Input: part model. Units: mm. Frame: model coordinates. Face numbers are marked on the shaded views. A direction names the side the tool comes from. Round coordinates to 2 decimals unless told otherwise and drop trailing zeros. Loops run counter-clockwise (first coordinate to the right, second up) from the corner with the lowest first, then second, coordinate; pieces in that order, holes last. Notation, with made-up numbers: (-35.75, 37.25) -> (21.25, 37.25) arc R30 cw to (21.25, 73.25) -> close; hole circle Ø8 at (76, -17). An arc over 180 degrees is marked (long way). Answer as a JSON object with one key per item and string values.
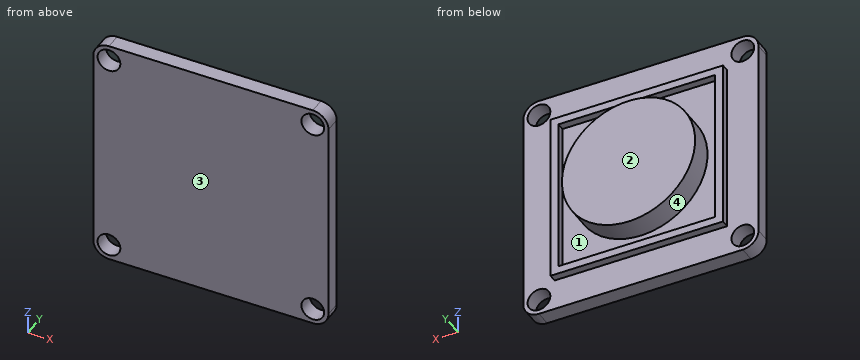
Autodesk Inventor part; units mm, degrees
ref_plane "YZ Plane" through (0, 0, 0) normal (1, 0, 0) x (0, 1, 0)
ref_plane "XZ Plane" through (0, 0, 0) normal (0, 1, 0) x (-1, 0, 0)
ref_plane "XY Plane" through (0, 0, 0) normal (0, 0, 1) x (1, 0, 0)
sketch "Boceto1" plane through (0, 0, 0) normal (0, 1, 0) x (-1, 0, 0)
  line L0 (-13, 15) -> (13, 15)
  line L1 (15, 13) -> (15, -13)
  line L2 (13, -15) -> (-13, -15)
  line L3 (-15, -13) -> (-15, 13)
  line L4 (-15, 15) -> (15, -15) construction
  line L5 (15, 15) -> (-15, -15) construction
  arc A0 (13, -15) -> (15, -13) centre (13, -13) ccw
  arc A1 (15, 13) -> (13, 15) centre (13, 13) ccw
  arc A2 (-13, 15) -> (-15, 13) centre (-13, 13) ccw
  arc A3 (-15, -13) -> (-13, -15) centre (-13, -13) ccw
  point P0 (0, 0)
  dimension "d0" = 30
  dimension "d1" = 30
  dimension "d2" = 2
extrude "Extrusión1" add sketch "Boceto1" along normal blind 2
sketch "Boceto2" plane through (0, 2, 0) normal (0, 1, 0) x (1, 0, 0)
  circle A0 centre (0, 0) radius 8.5
  dimension "d5" = 17
extrude "Extrusión2" add sketch "Boceto2" along normal blind 3
sketch "Boceto3" plane through (0, 2, 0) normal (0, 1, 0) x (1, 0, 0)
  line L0 (10, -10) -> (-10, -10)
  line L1 (-10, -10) -> (-10, 10)
  line L2 (-10, 10) -> (10, 10)
  line L3 (10, 10) -> (10, -10)
  line L4 (10, -10) -> (-10, 10) construction
  line L5 (-10, -10) -> (10, 10) construction
  line L6 (11, -11) -> (-11, -11)
  line L7 (-11, -11) -> (-11, 11)
  line L8 (-11, 11) -> (11, 11)
  line L9 (11, 11) -> (11, -11)
  line L10 (11, -11) -> (-11, 11) construction
  line L11 (-11, -11) -> (11, 11) construction
  point P0 (0, 0)
  dimension "d8" = 1
  dimension "d9" = 1
  dimension "d10" = 10
  dimension "d11" = 10
extrude "Extrusión3" add sketch "Boceto3" along normal blind 1
sketch "Boceto4" plane through (0, 0, 0) normal (0, -1, 0) x (1, 0, 0)
  point P0 (13, -13)
  point P1 (-13, -13)
hole "Agujero1" at (13, 0, -13) at (-13, 0, -13) direction (0, 1, 0) diameter 2.9 end through all
sketch "Boceto5" plane through (0, 0, 0) normal (0, -1, 0) x (1, 0, 0)
  point P0 (-13, 13)
hole "Agujero2" at (-13, 0, 13) direction (0, 1, 0) diameter 2.9 end through all
sketch "Boceto6" plane through (0, 0, 0) normal (0, -1, 0) x (1, 0, 0)
  point P0 (13, 13)
hole "Agujero3" at (13, 0, 13) direction (0, 1, 0) diameter 2.9 end through all
properties part number "Tapa trasera" material "Plástico PET"
1) Section C-C, the plane z = 0. Output: boundary loops of the cut face in (x, y).
Output:
{"outline": "(-15, 0) -> (15, 0) -> (15, 2) -> (11, 2) -> (11, 3) -> (10, 3) -> (10, 2) -> (8.5, 2) -> (8.5, 5) -> (-8.5, 5) -> (-8.5, 2) -> (-10, 2) -> (-10, 3) -> (-11, 3) -> (-11, 2) -> (-15, 2) -> close"}
2) Section B-B, the plane x = 0. Output: boundary loops of the cut face in (y, z).
Output:
{"outline": "(0, -15) -> (2, -15) -> (2, -11) -> (3, -11) -> (3, -10) -> (2, -10) -> (2, -8.5) -> (5, -8.5) -> (5, 8.5) -> (2, 8.5) -> (2, 10) -> (3, 10) -> (3, 11) -> (2, 11) -> (2, 15) -> (0, 15) -> close"}
3) Section A-A, the plane y = 2.65. Output: boundary loops of the cut face in (x, z), plus the area to 3 significant figures.
Output:
{"outline": "(-11, -11) -> (11, -11) -> (11, 11) -> (-11, 11) -> close; circle Ø17 at (0, 0); hole (-10, -10) -> (10, -10) -> (10, 10) -> (-10, 10) -> close", "area": "311 mm^2"}
4) Reachability of the marked faces 1 and 2 from +Z, -Z, +X, -X, +Y, -Y: full face, straight path, thin tool, end or side. Return the list, or none.
Output:
{"face 1": "+Y", "face 2": "+Z, -Z, +X, -X, +Y"}
5) Draft query along X for the marked faces 3 and 4. Return one class per face: +X half, -X half, draft (parallel to the pull), parting line (faces both ways), or undercut.
Output:
{"face 3": "draft", "face 4": "undercut"}
6) Contact query for flat-ended pins moving along their axis: P1, Ø2.5, axis at x = 13, z = -13, coming from the +Y side; P2, Ø2, axis at y = 3.5, z = -2, coming from the -X side; P3, Ø3, axis at x = -11.5, z = 2, coming from the +Y side. Output: stop coordinate, or through.
Output:
{"P1": "passes through", "P2": "stops at x = -11", "P3": "stops at y = 3"}
7) Ray query, probe 1 along Z at (x, y) = (-13, 1.5); probe 2 along Z at (x, y) = (-9.5, 2.8). Return the intervals inside material, ascending.
Output:
{"probe 1": "z = -15 to -14.45, -11.55 to 11.55, 14.45 to 15", "probe 2": "z = -11 to -10, 10 to 11"}
